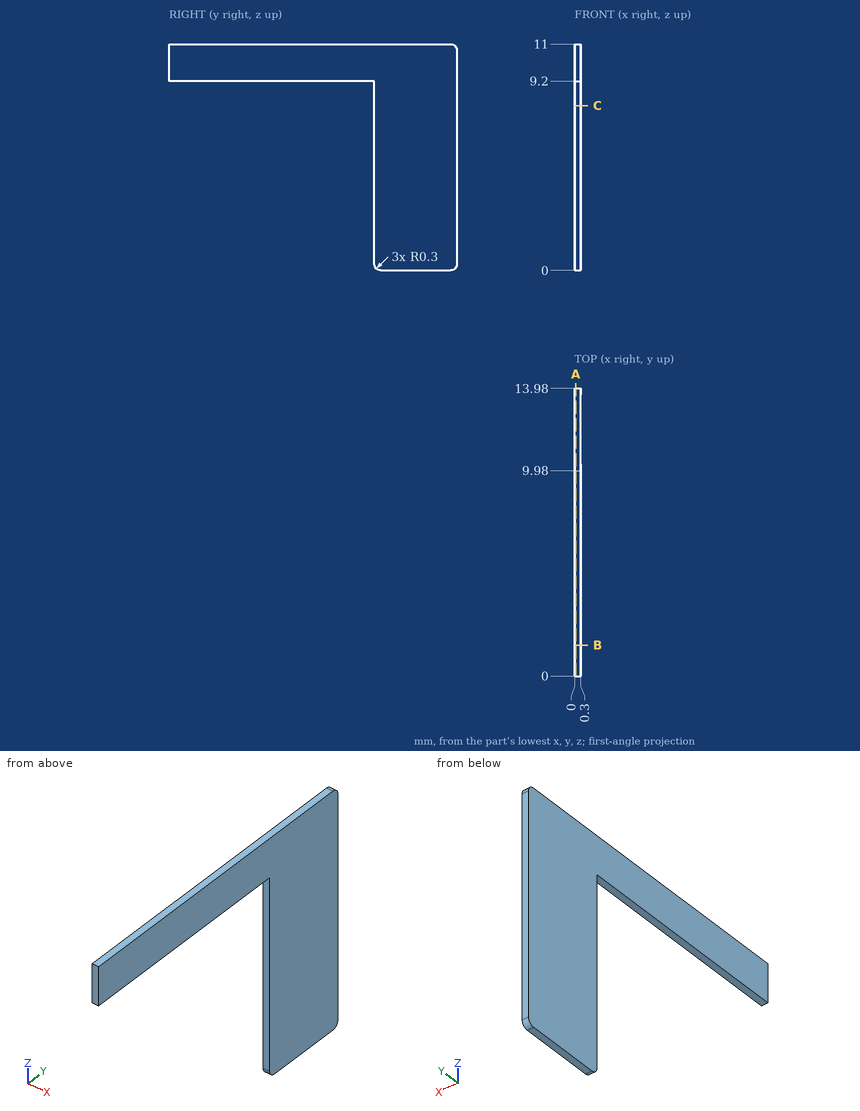
Study the drawing (mm; zero at the part's minimum x, y, z) and answer. Give positions to 0.01 mm unless a question says otherwise; leave off trailing zeros. Order: outer loops, then holes, each group sorted by start corner. A loop starts at its lowest first (then second) coordinate and runs counter-clockwise, first axis right, second up. Notation, with made-up numbers: (52.25, 80) - (95.25, 80) arc R14 ccw to (95.25, 95) - close; hole circle Ø5 at (18.25, 49.5). An arc over 180 degrees is marked (long way). Answer in a Markdown table with one row per item. Add a question column.
Q1. The part is cut by section B-B (y = 1.5). Determine the outline of the cut face in (x, z).
Q2. Find the intervals of material crossed by line 1 along Y through (x, z) = (0.2, 8.25); line 2 along Z through (x, y) = (0.2, 6.75), in increasing order. Write a range as [from, to].
Q3. The part is cut by section C-C (z = 8). Determine the outline of the cut face in (x, y), then the cut area to 3 significant figures.
Q4. The part is cut by section A-A (x = 0.05). Determine the outline of the cut face in (y, z), then the cut area to 3 significant figures.
Determined:
| question | item | result |
|---|---|---|
| 1 | outline | (0, 9.2) - (0.3, 9.2) - (0.3, 11) - (0, 11) - close |
| 2 | line 1 | y = [9.98, 13.98] |
| 2 | line 2 | z = [9.2, 11] |
| 3 | outline | (0, 9.98) - (0.3, 9.98) - (0.3, 13.98) - (0, 13.98) - close |
| 3 | area | 1.20 mm² |
| 4 | outline | (0, 9.2) - (9.98, 9.2) - (9.98, 0.3) arc R0.3 ccw to (10.28, 0) - (13.68, 0) arc R0.3 ccw to (13.98, 0.3) - (13.98, 10.7) arc R0.3 ccw to (13.68, 11) - (0, 11) - close |
| 4 | area | 61.9 mm² |
